Build history of the part. All positions in model axes, mm. Give positions to 0.01 mm unless a question says otherwise; leave off trailing zeros. Write each loop counter-clockwise with the first axis right and the second up, starting at its lowest first coordinate (ties: lowest second). Pieces come first, ordered by that corner, then holes.
Autodesk Fusion 360 part; units mm, degrees
sketch "Sketch1" plane through (0, 0, 0) normal (0, 1, 0) x (1, 0, 0)
  line L0 (25, 0) -> (0, -5)
  line L1 (25, 0) -> (0, 5)
  arc A0 (-3, -5) -> (0, -5) centre (-1.5, -4.5) ccw
  arc A1 (0, 5) -> (-3, 5) centre (-1.5, 4.5) ccw
  line L2 (-3, -5) -> (-3, 5)
  dimension "d1" = 3
extrude "Extrude1" add sketch "Sketch1" along normal blind 10
fillet "Fillet1" radius 1 5 edges at (12.5, 10, 2.5) (12.5, 10, -2.5) (-1.5, 10, 6.0811) (-3, 10, 0) (-1.5, 10, -6.0811)
fillet "Fillet2" radius 1 5 edges at (12.5, 0, 2.5) (-1.5, 0, 6.0811) (-3, 0, 0) (-1.5, 0, -6.0811) (12.5, 0, -2.5)
(1) Probe line 1 (Z direction, x = 2, y = 9.75); line 2 (Z direction, x = 8.5, y = 9); line 3 (Y direction, x = 4.5, z = -3.25). List the from-to ranges inside material, lowest first.
(2) Drop flat-ended pins along their axis: pin 1 (3 mm diameter, centred on x = 10.5, y = 9, fed in from +Z); pin 2 (2 mm diameter, centred on x = 0.5, y = 7.5, fed in from -Z); pin 3 (1.5 mm diameter, centred on x = 14.5, y = 8, fed in from -Z). Give the stop position or say it passes through.
(3) Saw through at A-A, the plane y = 4. List the corners of the cut face in (x, z), plus the area to 3 significant figures.
Computed values:
1. line 1: z = -4.25 to 4.25
1. line 2: z = -3.3 to 3.3
1. line 3: y = 0.01 to 9.99
2. pin 1: stops at z = 3.2
2. pin 2: stops at z = -5.72
2. pin 3: stops at z = -2.25
3. outline: (-3, -5) arc R1.58 ccw to (0, -5) - (25, 0) - (0, 5) arc R1.58 ccw to (-3, 5) - close
3. area: 160 mm2
